Read the model definition and answer for the solid it produces. Units are mm, in the model's axes. A direction names the side the tool comes from. Give positions to 0.01 mm unless a question says otherwise; leave off trailing zeros. Loops run counter-clockwise (first coordinate to the right, second up) from the corner with the lowest first, then second, coordinate; pieces in that order, holes last. Notation, with made-up numbers: (74, 83.25) - (123, 83.25) arc R12 cw to (123, 89.25) - close; hole circle Ø8 at (-19, -26). An arc over 180 degrees is marked (long way). Write each question's results on one line, items separated by ' | '. Start each with the question number.
Q1. Determine the mould class of faces 6 (the flat face through (96, -3, 37)), 7 (the flat face through (92.5, 4.3, 33.5)), 8 (the flat face through (73, 2, 93)) for opening direction Z: +Z half, -Z half, draft (parallel to the pull), parting line (faces both ways), or undercut.
Q2. For faces 1 (the flat face through (73, 2, 37)), 2 (the flat face through (96, -3, 93)), 3 (the flat face through (96, 7, 37)), 4 (the flat face through (92.5, 0.7, 96.5)), 5 (the flat face through (96, -5, 33)), determine the directions among +Z, -Z, +X, -X, +Y, -Y from which every point of the face is accessible in a straight line to the end or side of a thin tool.
Q3. Given pin 1 (2 mm diameter, centred on x = 67.5, z = 79.5, fed in from +Y); pin 2 (1.5 mm diameter, centred on x = 65.5, y = 2, fed in from -Z); pin 3 (8 mm diameter, centred on x = 83.5, y = -3.5, fed in from +Z), each flat-ended and moving along its own axis, determine where each tip first touches the part or whether it passes through.
Q4. The part is cut by section C-C, the plane x = 68.5. Write down the section's boundary in (y, z).
Q5. The part is cut by section B-B, the plane y = -2.5. Write down the section's boundary in (x, z), plus the area to 3 significant figures.
Q6. The part is cut by section D-D, the plane z = 85.5. Write down the section's boundary in (x, y), plus the area to 4 significant figures.
Q7. The part is cut by section A-A, the plane z = 33.5. Write down the section's boundary in (x, y), plus the area to 3 significant figures.
Q8. Find the intervals of material crossed by line 1 (Z direction, x = 95.5, y = 5.5); line 2 (Y direction, x = 98.5, z = 96.5); line 3 (Y direction, x = 97.5, z = 40.5), in increasing order. Write a range as from..to.
```python
from build123d import *

# Parameters (mm, degrees)
SKETCH_1_W          = 100
SKETCH_1_H          = 100
EXTRUDE_1_DEPTH     = 5
SKETCH_2_W          = 30
SKETCH_2_H          = 5
CUT_EXTRUDE_1_DEPTH = 100
CUT_EXTRUDE_2_DEPTH = 5
SKETCH_4_W          = 39
SKETCH_4_H          = 7
CUT_EXTRUDE_3_DEPTH = 5
SKETCH_5_W          = 7.5
SKETCH_5_H          = 5
EXTRUDE_2_DEPTH     = 70
SKETCH_6_W          = 56
SKETCH_6_H          = 5
CUT_EXTRUDE_5_DEPTH = 7.5
SKETCH_7_W          = 7
SKETCH_7_H          = 5
EXTRUDE_3_DEPTH     = 7.5
CUT_EXTRUDE_6_DEPTH = 7.5


with BuildPart() as part:
    # 草图1 → 凸台-拉伸1 (new body)
    with BuildSketch(Plane(origin=(0, 0, 0), x_dir=(1, 0, 0), z_dir=(0, 1, 0))):
        with Locations((50, -50)):
            Rectangle(SKETCH_1_W, SKETCH_1_H)
    extrude(amount=EXTRUDE_1_DEPTH)

    # 草图2 → 切除-拉伸1 (cut)
    with BuildSketch(Plane.ZY):
        with Locations((15, 2.5)):
            Rectangle(SKETCH_2_W, SKETCH_2_H)
    extrude(amount=-CUT_EXTRUDE_1_DEPTH, mode=Mode.SUBTRACT)

    # 草图3 → 切除-拉伸2 (cut)
    with BuildSketch(Plane.XZ):
        Polygon((53.5, 43.5), (53.5, 30), (0, 30), (0, 100), (53.5, 100), align=None)
    extrude(amount=-CUT_EXTRUDE_2_DEPTH, mode=Mode.SUBTRACT)

    # 草图4 → 切除-拉伸3 (cut)
    with BuildSketch(Plane.XZ):
        with Locations((73, 33.5)):
            Rectangle(SKETCH_4_W, SKETCH_4_H)
        with Locations((73, 96.5)):
            Rectangle(SKETCH_4_W, SKETCH_4_H)
    extrude(amount=-CUT_EXTRUDE_3_DEPTH, mode=Mode.SUBTRACT)

    # 草图5 → 凸台-拉伸2 (add)
    with BuildSketch(Plane(origin=(0, 0, 30), x_dir=(-1, 0, 0), z_dir=(0, 0, -1))):
        with Locations((-96.25, 7.5)):
            Rectangle(SKETCH_5_W, SKETCH_5_H)
    extrude(amount=-EXTRUDE_2_DEPTH)

    # 草图6 → 切除-拉伸5 (cut)
    with BuildSketch(Plane.ZY.offset(-92.5)):
        with Locations((65, 7.5)):
            Rectangle(SKETCH_6_W, SKETCH_6_H)
    extrude(amount=-CUT_EXTRUDE_5_DEPTH, mode=Mode.SUBTRACT)

    # 草图7 → 凸台-拉伸3 (add)
    with BuildSketch(Plane.ZY.offset(-92.5)):
        with Locations((33.5, -2.5)):
            Rectangle(SKETCH_7_W, SKETCH_7_H)
        with Locations((96.5, -2.5)):
            Rectangle(SKETCH_7_W, SKETCH_7_H)
    extrude(amount=-EXTRUDE_3_DEPTH)

    # 草图8 → 切除-拉伸6 (cut)
    with BuildSketch(Plane.ZY.offset(-92.5)):
        with BuildLine():
            ThreePointArc((32.198026446, 3.42998111), (32.57001889, 1.198026446), (34.801973554, 1.57001889))
            Line((34.801973554, 1.57001889), (32.198026446, 3.42998111))
        make_face()
        with BuildLine():
            Line((32.198026446, 3.42998111), (34.801973554, 1.57001889))
            ThreePointArc((34.801973554, 1.57001889), (35.023672814, 2.01171611), (35.1, 2.5))
            ThreePointArc((35.1, 2.5), (33.98828389, 4.023672814), (32.198026446, 3.42998111))
        make_face()
        with BuildLine():
            ThreePointArc((98.1, 2.5), (96.98828389, 4.023672814), (95.198026446, 3.42998111))
            Line((95.198026446, 3.42998111), (97.801973554, 1.57001889))
            ThreePointArc((97.801973554, 1.57001889), (98.023672814, 2.01171611), (98.1, 2.5))
        make_face()
        with BuildLine():
            Line((97.801973554, 1.57001889), (95.198026446, 3.42998111))
            ThreePointArc((95.198026446, 3.42998111), (95.57001889, 1.198026446), (97.801973554, 1.57001889))
        make_face()
    extrude(amount=-CUT_EXTRUDE_6_DEPTH, mode=Mode.SUBTRACT)


solid = part.part
```
Check sheet entries:
1) face 6: undercut | face 7: draft | face 8: +Z half
2) face 1: -Z, -X, +Y, -Y | face 2: +X, -X, -Y | face 3: +X, -X, +Y | face 4: +Z, -X, +Y, -Y | face 5: +Z, -Z, +X, -X, -Y
3) pin 1: stops at y = 5 | pin 2: stops at z = 37 | pin 3: stops at z = 93
4) outline: (0, 37) - (5, 37) - (5, 93) - (0, 93) - close
5) outline: (92.5, 30) - (100, 30) - (100, 37) - (92.5, 37) - close; (92.5, 93) - (100, 93) - (100, 100) - (92.5, 100) - close | area: 105 mm^2
6) outline: (53.5, 0) - (100, 0) - (100, 5) - (53.5, 5) - close | area: 232.5 mm^2
7) outline: (92.5, -5) - (100, -5) - (100, 0.9) - (92.5, 0.9) - close; (92.5, 4.1) - (100, 4.1) - (100, 10) - (92.5, 10) - close | area: 88.5 mm^2
8) line 1: z = 30..37, 93..100 | line 2: y = -5..0.9, 4.1..10 | line 3: y = 0..5
